```python
from build123d import *

# Parameters (mm, degrees)
F0_W      = 72.898
F0_H      = 72.898
F1_DEPTH  = 76.2
F2_R      = 5.08
F3_R      = 6.35
F4_DEPTH  = 5.08
F6_DEPTH  = 5.08
F7_R      = 6.35
F8_DEPTH  = 5.08
F9_R      = 6.35
F10_DEPTH = 5.08
F11_R     = 6.35
F12_DEPTH = 5.08
F13_R     = 6.35
F14_DEPTH = 5.08


with BuildPart() as f1:
    # F0 (on Top) → F1 (new body)
    with BuildSketch(Plane.XY):
        with Locations((-56.9363877252, 21.6006250121)):
            Rectangle(F0_W, F0_H)
    extrude(amount=F1_DEPTH)

    # F2
    f2_edges = [f1.edges().sort_by_distance(p)[0] for p in [
        (-20.487388, 21.600625, 76.2),
        (-93.385388, 58.049625, 38.1),
        (-56.936388, 58.049625, 0),
        (-20.487388, 58.049625, 38.1),
        (-20.487388, 21.600625, 0),
        (-56.936388, 58.049625, 76.2),
        (-20.487388, -14.848375, 38.1),
        (-93.385388, 21.600625, 0),
        (-56.936388, -14.848375, 0),
        (-56.936388, -14.848375, 76.2),
        (-93.385388, -14.848375, 38.1),
        (-93.385388, 21.600625, 76.2),
    ]]
    fillet(f2_edges, radius=F2_R)

    # F3 (on face) → F4 (cut)
    with BuildSketch(Plane.XY.offset(76.2)):
        with Locations((-56.9363877252, 21.6006250121)):
            Circle(F3_R)
    extrude(amount=-F4_DEPTH, mode=Mode.SUBTRACT)

    # F5 (on face) → F6 (cut)
    with BuildSketch(Plane(origin=(0, 0, 0), x_dir=(1, 0, 0), z_dir=(0, 0, -1))):
        with BuildLine():
            Line((-71.9999372959, -8.0116250121), (-71.9999372959, 4.6883749879))
            ThreePointArc((-71.9999372959, 4.6883749879), (-78.3499372959, -1.6616250121), (-71.9999372959, -8.0116250121))
        make_face()
        with BuildLine():
            ThreePointArc((-65.6499372959, -1.6616250121), (-67.5098092354, 2.8285030485), (-71.9999372959, 4.6883749879))
            Line((-71.9999372959, 4.6883749879), (-71.9999372959, -8.0116250121))
            ThreePointArc((-71.9999372959, -8.0116250121), (-67.5098092354, -6.1517530726), (-65.6499372959, -1.6616250121))
        make_face()
        with BuildLine():
            ThreePointArc((-71.9999372959, -15.2506250121), (-78.3499372959, -21.6006250121), (-71.9999372959, -27.9506250121))
            Line((-71.9999372959, -27.9506250121), (-71.9999372959, -15.2506250121))
        make_face()
        with BuildLine():
            Line((-71.9999372959, -15.2506250121), (-71.9999372959, -27.9506250121))
            ThreePointArc((-71.9999372959, -27.9506250121), (-67.5098092354, -26.0907530726), (-65.6499372959, -21.6006250121))
            ThreePointArc((-65.6499372959, -21.6006250121), (-67.5098092354, -17.1104969515), (-71.9999372959, -15.2506250121))
        make_face()
        with BuildLine():
            ThreePointArc((-71.9999372959, -35.1896250121), (-78.3499372959, -41.5396250121), (-71.9999372959, -47.8896250121))
            Line((-71.9999372959, -47.8896250121), (-71.9999372959, -35.1896250121))
        make_face()
        with BuildLine():
            ThreePointArc((-40.0320217013, -35.1896250121), (-46.3820217013, -41.5396250121), (-40.0320217013, -47.8896250121))
            Line((-40.0320217013, -47.8896250121), (-40.0320217013, -35.1896250121))
        make_face()
        with BuildLine():
            Line((-40.0320217013, -35.1896250121), (-40.0320217013, -47.8896250121))
            ThreePointArc((-40.0320217013, -47.8896250121), (-35.5418936408, -46.0297530726), (-33.6820217013, -41.5396250121))
            ThreePointArc((-33.6820217013, -41.5396250121), (-35.5418936408, -37.0494969515), (-40.0320217013, -35.1896250121))
        make_face()
        with BuildLine():
            ThreePointArc((-40.0320217013, -15.2506250121), (-46.3820217013, -21.6006250121), (-40.0320217013, -27.9506250121))
            Line((-40.0320217013, -27.9506250121), (-40.0320217013, -15.2506250121))
        make_face()
        with BuildLine():
            Line((-40.0320217013, -15.2506250121), (-40.0320217013, -27.9506250121))
            ThreePointArc((-40.0320217013, -27.9506250121), (-35.5418936408, -26.0907530726), (-33.6820217013, -21.6006250121))
            ThreePointArc((-33.6820217013, -21.6006250121), (-35.5418936408, -17.1104969515), (-40.0320217013, -15.2506250121))
        make_face()
        with BuildLine():
            Line((-40.0320217013, -8.0116250121), (-40.0320217013, 4.6883749879))
            ThreePointArc((-40.0320217013, 4.6883749879), (-46.3820217013, -1.6616250121), (-40.0320217013, -8.0116250121))
        make_face()
        with BuildLine():
            ThreePointArc((-33.6820217013, -1.6616250121), (-35.5418936408, 2.8285030485), (-40.0320217013, 4.6883749879))
            Line((-40.0320217013, 4.6883749879), (-40.0320217013, -8.0116250121))
            ThreePointArc((-40.0320217013, -8.0116250121), (-35.5418936408, -6.1517530726), (-33.6820217013, -1.6616250121))
        make_face()
        with BuildLine():
            Line((-71.9999372959, -35.1896250121), (-71.9999372959, -47.8896250121))
            ThreePointArc((-71.9999372959, -47.8896250121), (-67.5098092354, -46.0297530726), (-65.6499372959, -41.5396250121))
            ThreePointArc((-65.6499372959, -41.5396250121), (-67.5098092354, -37.0494969515), (-71.9999372959, -35.1896250121))
        make_face()
    extrude(amount=-F6_DEPTH, mode=Mode.SUBTRACT)

    # F7 (on face) → F8 (cut)
    with BuildSketch(Plane.YZ.offset(-20.4873877252)):
        with Locations((39.1023317684, 56.5228492172)):
            Circle(F7_R)
        with Locations((4.5328344803, 20.1339047034)):
            Circle(F7_R)
    extrude(amount=-F8_DEPTH, mode=Mode.SUBTRACT)

    # F9 (on face) → F10 (cut)
    with BuildSketch(Plane(origin=(0, 58.0496250121, 0), x_dir=(-1, 0, 0), z_dir=(0, 1, 0))):
        with Locations((75.1341481229, 57.2555372607)):
            Circle(F9_R)
        with Locations((56.9363877252, 38.1)):
            Circle(F9_R)
        with Locations((38.2840325717, 18.4659419437)):
            Circle(F9_R)
    extrude(amount=-F10_DEPTH, mode=Mode.SUBTRACT)

    # F11 (on face) → F12 (cut)
    with BuildSketch(Plane.XZ.offset(14.8483749879)):
        with Locations((-74.3611752987, 55.96582219)):
            Circle(F11_R)
        with Locations((-36.3990627229, 55.96582219)):
            Circle(F11_R)
        with Locations((-36.3990627229, 19.5222850889)):
            Circle(F11_R)
        with Locations((-74.3611752987, 19.5222850889)):
            Circle(F11_R)
    extrude(amount=-F12_DEPTH, mode=Mode.SUBTRACT)

    # F13 (on face) → F14 (cut)
    with BuildSketch(Plane(origin=(-93.3853877252, 0, 0), x_dir=(0, -1, 0), z_dir=(-1, 0, 0))):
        with Locations((-41.9357791543, 54.5396991074)):
            Circle(F13_R)
        with Locations((-21.6006250121, 40.0424264371)):
            Circle(F13_R)
        with Locations((-0.0511793769, 54.5396991074)):
            Circle(F13_R)
        with Locations((-0.0511793769, 20.7625031471)):
            Circle(F13_R)
        with Locations((-41.9357791543, 20.7625031471)):
            Circle(F13_R)
    extrude(amount=-F14_DEPTH, mode=Mode.SUBTRACT)


solid = f1.part
```
Geometry check sheet. Reference: the model listing, model coordinates, mm. A direction names the side the tool comes from. Round coordinates to 2 decimals unless told otherwise and drop trailing zeros. Order: outer loops, then holes, each group sorted by start corner. A loop starts at its lowest first (then second) coordinate and runs counter-clockwise, first axis right, second up. Notation, with made-up numbers: (13.25, 52.5) -> (70.25, 52.5) arc R13 ccw to (70.25, 59.5) -> close; hole circle Ø7 at (-26, -36). An arc over 180 degrees is marked (long way). Return JSON: item names as keys, results as strings. Group by question number.
Q1. Release check for a two-part mould opening along X. For faces 4 (the cylindrical face through (-21.936, 22.04, 1.528)), 5 (the flat face through (-74, -9.768, 56)), 6 (the cylindrical face through (-91.94, 22.04, 74.67)) record: released by +X, released by -X, zero draft, split by the parting line, or undercut.
Q2. Gauge pin test, flat ends, axial feed: pin 1 (7.5 mm diameter, centred on x = -38.28, z = 18.47, fed in from +Y); pin 2 (4 mm diameter, centred on x = -75.5, z = 54, fed in from -Y); pin 3 (4 mm diameter, centred on x = -42, y = 41, fed in from -Z). Record the tip position at first contact, or that the pin passes through.
Q3. Material ranges on probe 1 along X at (y, z) = (6, 71.5); probe 2 along Y at (x, z) = (-79, 16.5); probe 3 along X at (y, z) = (53.5, 63), recorded low to high. Write a range as from..to.
Q4. Section check A-A, the plane z = 38.1. Record the boundary of the cut face in (x, y) (3 decimals).
Q5. Tool access check on faces 1 (the flat face through (-36, -9.768, 20)), 2 (the cylindrical face through (-90.881, 0.878, 60.836)), 3 (the cylindrical face through (-51.897, 55.545, 34.236)). Record the directions out of +Z, -Z, +X, -X, +Y, -Y that give a thin tool (end or side, any length) a straight path to the whole face; none if there is none.
Numbers:
{
 "1": {"face 4": "released by +X", "face 5": "undercut", "face 6": "released by -X"},
 "2": {"pin 1": "y = 52.97", "pin 2": "y = -9.77", "pin 3": "z = 5.08"},
 "3": {"probe 1": "-93.37..-20.5", "probe 2": "-9.77..58.05", "probe 3": "-93.36..-77.84, -72.43..-20.52"},
 "4": {"outline": "(-93.385, -9.768) arc R5.08 ccw to (-88.305, -14.848) -> (-25.567, -14.848) arc R5.08 ccw to (-20.487, -9.768) -> (-20.487, 52.97) arc R5.08 ccw to (-25.567, 58.05) -> (-50.586, 58.05) -> (-50.586, 52.97) -> (-63.286, 52.97) -> (-63.286, 58.05) -> (-88.305, 58.05) arc R5.08 ccw to (-93.385, 52.97) -> (-93.385, 27.646) -> (-88.305, 27.646) -> (-88.305, 15.555) -> (-93.385, 15.555) -> close"},
 "5": {"face 1": "-Y", "face 2": "-X", "face 3": "+Y"}
}
